```python
from build123d import *

# Parameters (mm, degrees)
F1_DEPTH  = 9
F5_W      = 2
F5_H      = 2
F6_DEPTH  = 8
F7_DEPTH  = 2
F5_H_2    = 4.65
F5_H_3    = 2.7
F8_DEPTH  = 100
F9_W      = 224.7
F9_H      = 51.4
F9_W_2    = 220.7
F9_H_2    = 47.4
F10_DEPTH = 2


with BuildPart() as f1:
    # F0 (on Top) → F1 (new body)
    with BuildSketch(Plane.XY):
        Polygon((-23.7, -23.7), (23.7, -23.7), (23.7, 0), (21.2, 0), (21.2, -21.2), (-21.2, -21.2), (-21.2, -5), (-23.7, -5), align=None)
        Polygon((21.2, 0), (23.7, 0), (23.7, 23.7), (-23.7, 23.7), (-23.7, 5), (-21.2, 5), (-21.2, 21.2), (21.2, 21.2), align=None)
    extrude(amount=F1_DEPTH)



with BuildPart() as f6:
    # F5 (on line) → F6 (new body)
    with BuildSketch(Plane.XY.offset(100)):
        Polygon((195, -4.65), (177, -4.65), (177, -6.65), (197, -6.65), (197, -2.7), (195, -2.7), align=None)
        with Locations((176, -5.65)):
            Rectangle(F5_W, F5_H)
    extrude(amount=F6_DEPTH)



with BuildPart() as f6b:
    # F5 (on line) → F6, piece 2 (new body)
    with BuildSketch(Plane.XY.offset(100)):
        Polygon((177, 6.65), (177, 4.65), (195, 4.65), (195, 2.7), (197, 2.7), (197, 6.65), align=None)
        with Locations((176, 5.65)):
            Rectangle(F5_W, F5_H)
    extrude(amount=F6_DEPTH)


with BuildPart() as f6_1:
    add(f6.part)

    add(f6b.part)  # F7 merges F6b
    # F5 (on line) → F7 (join)
    with BuildSketch(Plane.XY.offset(100)):
        Polygon((177, 4.65), (177, 0), (177, -4.65), (195, -4.65), (195, -2.7), (195, 0), (195, 2.7), (195, 4.65), align=None)
    extrude(amount=-F7_DEPTH)

    # F5 (on line) → F8 (join)
    with BuildSketch(Plane.XY.offset(100)):
        Polygon((195, -4.65), (177, -4.65), (177, -6.65), (197, -6.65), (197, -2.7), (195, -2.7), align=None)
        with Locations((176, -5.65)):
            Rectangle(F5_W, F5_H)
        with Locations((176, -2.325)):
            Rectangle(F5_W, F5_H_2)
        with Locations((176, 2.325)):
            Rectangle(F5_W, F5_H_2)
        with Locations((176, 5.65)):
            Rectangle(F5_W, F5_H)
        Polygon((177, 6.65), (177, 4.65), (195, 4.65), (195, 2.7), (197, 2.7), (197, 6.65), align=None)
        with Locations((196, -1.35)):
            Rectangle(F5_W, F5_H_3)
        with Locations((196, 1.35)):
            Rectangle(F5_W, F5_H_3)
    extrude(amount=-F8_DEPTH)


with BuildPart() as f1_1:
    add(f1.part)

    add(f6_1.part)  # F10 merges F6
    # F9 (on Top) → F10 (join)
    with BuildSketch(Plane.XY):
        with Locations((86.65, 0)):
            Rectangle(F9_W, F9_H)
        with Locations((86.65, 0)):
            Rectangle(F9_W_2, F9_H_2, mode=Mode.SUBTRACT)
        with Locations((86.65, 0)):
            Rectangle(F9_W_2, F9_H_2)
    extrude(amount=-F10_DEPTH)


solid = f1_1.part
```
The model under review builds one solid part; all positions refer to its coordinate system, in mm. A direction names the side the tool comes from. Give positions to 0.01 mm unless a question says otherwise; leave off trailing zeros. Write each loop counter-clockwise with the first axis right and the second up, starting at its lowest first coordinate (ties: lowest second). Pieces come first, ordered by that corner, then holes. Notation, with made-up numbers: (-35.5, 24) -> (-12.5, 24) arc R16 ccw to (-12.5, 32) -> close; hole circle Ø5 at (-18, -19). An arc over 180 degrees is marked (long way). Put each result on its own line as item: value.
(1) For pin 1 Ø5.5 at (x, z) = (188, 72) entering from -Y; pin 2 Ø10.5 at (y, z) = (-1, 49) entering from -X; pin 3 Ø10 at (y, z) = (-13.5, 6.5) entering from +X; pin 4 Ø7 at (x, z) = (9, 2.5) entering from -Y, all flat-tipped, find the tip position at first contact; note any pin that passes through.
Results are:
pin 1: y = -6.65
pin 2: x = 175
pin 3: x = 23.7
pin 4: y = -25.7
(2) We need section B-B, the plane z = 78.5. Give the boundary of the cut face in (x, y).
Results are:
outline: (175, -6.65) -> (197, -6.65) -> (197, 6.65) -> (175, 6.65) -> close; hole (177, -4.65) -> (195, -4.65) -> (195, 4.65) -> (177, 4.65) -> close
(3) We need section A-A, the plane x = 4. Give the boundary of the cut face in (y, z).
Results are:
outline: (-25.7, -2) -> (25.7, -2) -> (25.7, 0) -> (23.7, 0) -> (23.7, 9) -> (21.2, 9) -> (21.2, 0) -> (-21.2, 0) -> (-21.2, 9) -> (-23.7, 9) -> (-23.7, 0) -> (-25.7, 0) -> close
(4) To check wall thickness, follow probe 1 along X at (y, z) = (4, 30.5); probe 2 along Z at (x, y) = (145, 13); probe 3 along X at (y, z) = (5, 80.5). State the ranges of each line that lie inside material, in increasing order. Write a range as from..to.
Results are:
probe 1: 175..177, 195..197
probe 2: -2..0
probe 3: 175..197
(5) The part is to be moulded in two halves that separate along Y. For faces 1 (the flat face through (186, 6.65, 55)), 2 (the flat face through (185, 4.65, 104)), 3 (the flat face through (186, -6.65, 55)), say which applies: pulls with the +Y half, pulls with the -Y half, needs draft (parallel to the pull), parting line crosses it, or undercut.
Results are:
face 1: pulls with the +Y half
face 2: undercut
face 3: pulls with the -Y half
(6) Tool access review of faces 4 (the flat face through (-23.7, 14, 4)), 5 (the flat face through (0, -23.7, 4)), 6 (the flat face through (186, -4.65, 50)), 7 (the flat face through (185, -4.65, 104)): name each direction out of +Z, -Z, +X, -X, +Y, -Y from which nothing blocks a thin tool from reaching the whole face with its end or side.
Results are:
face 4: +Z, -X, +Y, -Y
face 5: +Z, +X, -X, -Y
face 6: none
face 7: +Z, -X
(7) We need section D-D, the plane x = 121. Give the boundary of the cut face in (y, z), and give its area (3 significant figures).
Results are:
outline: (-25.7, -2) -> (25.7, -2) -> (25.7, 0) -> (-25.7, 0) -> close
area: 103 mm²
(8) We need section C-C, the plane y = 13. Give the boundary of the cut face in (x, z).
Results are:
outline: (-25.7, -2) -> (199, -2) -> (199, 0) -> (23.7, 0) -> (23.7, 9) -> (21.2, 9) -> (21.2, 0) -> (-21.2, 0) -> (-21.2, 9) -> (-23.7, 9) -> (-23.7, 0) -> (-25.7, 0) -> close
